from build123d import *

# Parameters (mm, degrees)
EXTRUDE1_DEPTH = 1.5875
CHAMFER1_SIZE  = 1.397


with BuildPart() as part:
    # Sketch1 → Extrude1 (new, symmetric)
    with BuildSketch(Plane.XY):
        Polygon((0, 0), (193.675, 0), (127, 203.2), (0, 203.2), (-127, 203.2), (-193.675, 0), align=None)
    extrude(amount=EXTRUDE1_DEPTH, both=True)

    # Chamfer1
    chamfer1_edges = [part.edges().sort_by_distance(p)[0] for p in [
        (160.3375, 101.6, 1.5875),
        (0, 203.2, 1.5875),
        (-160.3375, 101.6, 1.5875),
        (-160.3375, 101.6, -1.5875),
        (0, 203.2, -1.5875),
        (160.3375, 101.6, -1.5875),
    ]]
    chamfer(chamfer1_edges, length=CHAMFER1_SIZE)


solid = part.part
The listing builds one solid part. Answer for the finished solid, in the listing's coordinates (mm). Give positions to 0.01 mm unless a question says otherwise; leave off trailing zeros. Write each loop counter-clockwise with the first axis right and the second up, starting at its lowest first coordinate (ties: lowest second). Pieces come first, ordered by that corner, then holes. Notation, with made-up numbers: (-1.5, 5.5) - (31.5, 5.5) arc R31 ccw to (31.5, 29.5) - close; hole circle Ø7 at (-12.75, 2.25). An arc over 180 degrees is marked (long way). Use a Markdown table: item, result.
1. Section C-C on y = 21.5 is taken. Write down the section's boundary in (x, z), plus the area to 3 significant figures.
Values follow:
| item | result |
|---|---|
| outline | (-186.62, -0.19) - (-185.15, -1.59) - (185.15, -1.59) - (186.62, -0.19) - (186.62, 0.19) - (185.15, 1.59) - (-185.15, 1.59) - (-186.62, 0.19) - close |
| area | 1,180 mm² |
2. Section B-B on x = 150 is taken. Write down the section's boundary in (y, z), plus the area to 3 significant figures.
Values follow:
| item | result |
|---|---|
| outline | (0, -1.59) - (128.62, -1.59) - (133.1, -0.19) - (133.1, 0.19) - (128.62, 1.59) - (0, 1.59) - close |
| area | 416 mm² |
3. Section D-D on z = -0.75 is taken. Write down the section's boundary in (x, y), plus the area to 3 significant figures.
Values follow:
| item | result |
|---|---|
| outline | (-193.09, 0) - (193.09, 0) - (126.59, 202.64) - (-126.59, 202.64) - close |
| area | 64,800 mm² |
4. This flat-tipped pin is pushed along its axis until it touches: P1, Ø1.5, axis at x = 85.5, z = -1, coming from the +Y side. Where does it stop, or does it pass through?
Values follow:
| item | result |
|---|---|
| P1 | stops at y = 203.14 |
5. Find the intervals of material crossed by probe 1 along Y at (x, z) = (-7.5, 0.8); probe 2 along Y at (x, z) = (39, -0.4); probe 3 along X at (y, z) = (130, 0.3), in increasing order. Write a range as from..to.
Values follow:
| item | result |
|---|---|
| probe 1 | y = 0..202.59 |
| probe 2 | y = 0..202.99 |
| probe 3 | x = -150.9..150.9 |
6. Section A-A on y = 180 is taken. Write down the section's boundary in (x, z).
Values follow:
| item | result |
|---|---|
| outline | (-134.61, -0.19) - (-133.14, -1.59) - (133.14, -1.59) - (134.61, -0.19) - (134.61, 0.19) - (133.14, 1.59) - (-133.14, 1.59) - (-134.61, 0.19) - close |
